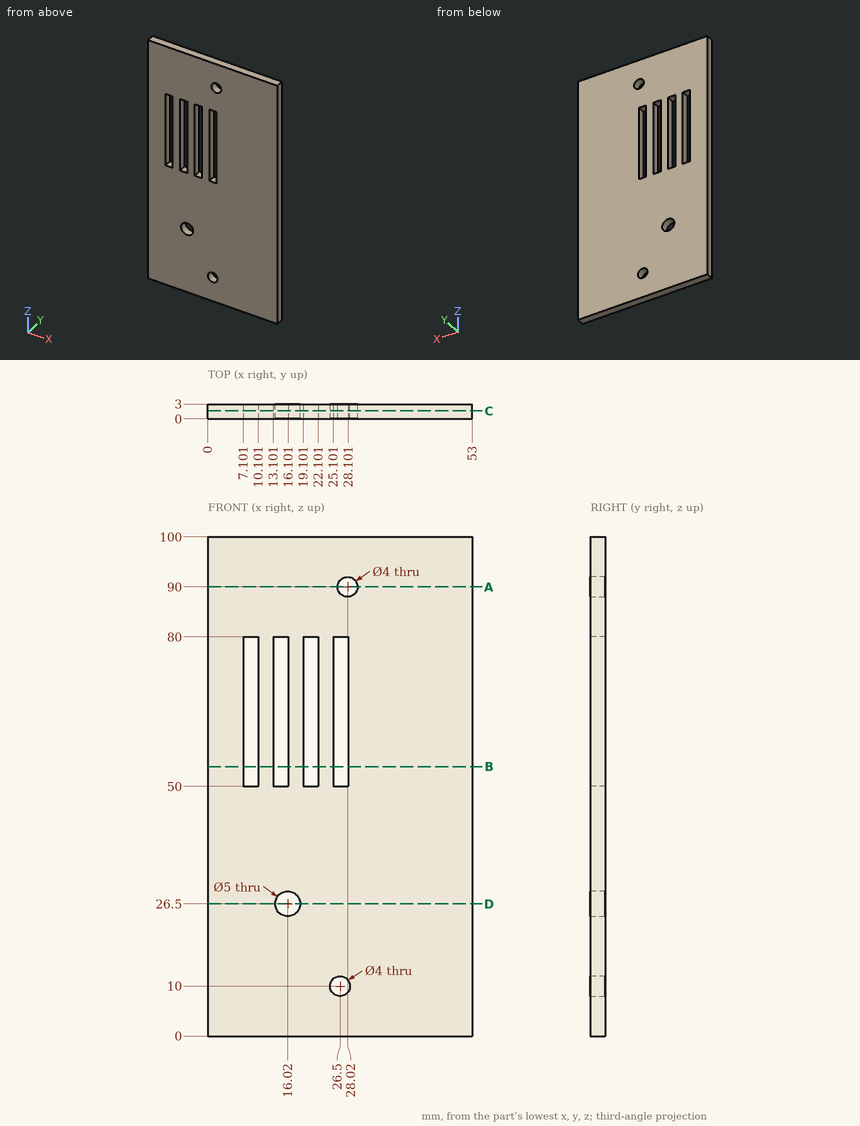
Source: three-view drawing plus pictorial views. Frame: mm from the lowest corner of the part. Round coordinates to 2 decimals unless told otherwise and drop trailing zeros. Loops run counter-clockwise (first coordinate to the right, second up) from the corner with the lowest first, then second, coordinate; pieces in that order, holes last.
Item 1: Section D-D, the plane z = 26.5. Output: boundary loops of the cut face in (x, y).
Checked values:
outline: (0, 0) - (13.52, 0) - (13.52, 3) - (0, 3) - close; (18.52, 0) - (53, 0) - (53, 3) - (18.52, 3) - close
Item 2: Line query: L1, parallel to X at y = 2.35, z = 60; L2, parallel to Z at x = 14.5, y = 2.65 (1 decimal); L3, parallel to X at y = 1.85, z = 10. Output: solid intervals per line, ascending.
Checked values:
L1: x = 0 to 7.1, 10.1 to 13.1, 16.1 to 19.1, 22.1 to 25.1, 28.1 to 53
L2: z = 0 to 24.5, 28.5 to 50, 80 to 100
L3: x = 0 to 24.5, 28.5 to 53
Item 3: Contact query for a flat-ended pin moving along its axis: P1, Ø4.5, axis at x = 16.02, z = 26.5, coming from the +Y side. Output: stop coordinate, or through.
Checked values:
P1: passes through
Item 4: Section A-A, the plane z = 90. Output: boundary loops of the cut face in (x, y).
Checked values:
outline: (0, 0) - (26.02, 0) - (26.02, 3) - (0, 3) - close; (30.02, 0) - (53, 0) - (53, 3) - (30.02, 3) - close
Item 5: Section B-B, the plane z = 54. Output: boundary loops of the cut face in (x, y).
Checked values:
outline: (0, 0) - (7.1, 0) - (7.1, 3) - (0, 3) - close; (10.1, 0) - (13.1, 0) - (13.1, 3) - (10.1, 3) - close; (16.1, 0) - (19.1, 0) - (19.1, 3) - (16.1, 3) - close; (22.1, 0) - (25.1, 0) - (25.1, 3) - (22.1, 3) - close; (28.1, 0) - (53, 0) - (53, 3) - (28.1, 3) - close
Item 6: Section C-C, the plane y = 1.6. Output: boundary loops of the cut face in (x, z).
Checked values:
outline: (0, 0) - (53, 0) - (53, 100) - (0, 100) - close; hole (7.1, 50) - (10.1, 50) - (10.1, 80) - (7.1, 80) - close; hole (13.1, 50) - (16.1, 50) - (16.1, 80) - (13.1, 80) - close; hole circle Ø5 at (16.02, 26.5); hole (19.1, 50) - (22.1, 50) - (22.1, 80) - (19.1, 80) - close; hole circle Ø4 at (26.5, 10); hole (25.1, 50) - (28.1, 50) - (28.1, 80) - (25.1, 80) - close; hole circle Ø4 at (28.02, 90)
